Could you check a few things on this model? Use its own coordinates, in mm. A direction names the side the tool comes from. Coordinates: 2 decimals unless noted, no trailing zeros. Order: outer loops, then holes, each group sorted by start corner. A loop starts at its lowest first (then second) coordinate and runs counter-clockwise, first axis right, second up. Notation, with made-up numbers: (1.5, 14.5) - (49.5, 14.5) arc R26 ccw to (49.5, 36.5) - close; hole circle Ø10 at (33, 2). An arc over 180 degrees is marked (long way). Answer as a JSON object with one key per item and string values. Group by question number.
(1) Which directions (+Z, -Z, +X, -X, +Y, -Y) give clear straight access to the entire face, cutting with the end or side of a thin tool? Please do faces 1 (the cylindrical face through (68.57, 14.45, -7.45)), 2 (the flat face through (62, 22, -80)), 3 (the flat face through (9, 24, -11)), 4 (the flat face through (29, 40, -2)).
(2) Please list where these lines run through material, in increasing order: probe 1 along Y at (x, z) = (116, -8) (3 decimals); probe 2 along Y at (x, z) = (70, -10) (3 decimals); probe 3 along X at (y, z) = (26.5, -68.5).
(3) We'd pull the mould along X, two halves only. Please class faces 5 (the flat face through (0, 22, -39)), 6 (the flat face through (62, 22, 0)), 7 (the flat face through (121, 24, -39)): pulls with the +X half, pulls with the -X half, needs draft (parallel to the pull), parting line crosses it, or undercut.
(4) Imagine slicing it at C-C, the plane z = -44.5. Write out the boundary of the cut face in (x, y).
(5) Imagine slicing it at A-A, the plane y = 9.5. Write out the boundary of the cut face in (x, z), and give its area (3 significant figures).
(6) Imagine slicing it at B-B, the plane x = 77.5. Write out the boundary of the cut face in (y, z), and give its area (3 significant figures).
(7) Will these pins go through, and if not, where does the flat tip stop? P1, Ø4, axis at x = 63.5, z = -37, coming from the +Y side; P2, Ø4.5, axis at y = 24.5, z = -1.5, coming from the -X side.
from build123d import *

# Parameters (mm, degrees)
BASE_SKETCH_W                   = 125
BASE_SKETCH_H                   = 80
BASE_EXTRUDE_DEPTH              = 4
WALL_BASE_SKETCH_W              = 125
WALL_BASE_SKETCH_H              = 80
WALL_BASE_SKETCH_W_2            = 117
WALL_BASE_SKETCH_H_2            = 72
WALL_BASE_EXTRUDE_DEPTH         = 40
SPEAKER_HOLE_SKETCH_W           = 28
SPEAKER_HOLE_SKETCH_H           = 32
SPEAKER_HOLE_DEPTH              = 7
SPEAKER_STANDOFFS_SKETCH_R      = 3.5
SPEAKER_STANDOFFS_SKETCH_R_2    = 1.5
SPEAKER_STANDOFFS_EXTRUDE_DEPTH = 7
M1_2X0_25_TAPPED_HOLE2_D        = 0.95
M1_2X0_25_TAPPED_HOLE2_DEPTH    = 3.15
M1_2X0_25_TAPPED_HOLE2_TIP      = 0.285408794


with BuildPart() as part:
    # base sketch → base extrude (new body)
    with BuildSketch(Plane(origin=(0, 0, 0), x_dir=(1, 0, 0), z_dir=(0, 1, 0))):
        with Locations((62.5, 40)):
            Rectangle(BASE_SKETCH_W, BASE_SKETCH_H)
    extrude(amount=BASE_EXTRUDE_DEPTH)

    # wall base sketch → wall base extrude (add)
    with BuildSketch(Plane(origin=(0, 4, 0), x_dir=(1, 0, 0), z_dir=(0, 1, 0))):
        with Locations((62.5, 40)):
            Rectangle(WALL_BASE_SKETCH_W, WALL_BASE_SKETCH_H)
        with Locations((62.5, 40)):
            Rectangle(WALL_BASE_SKETCH_W_2, WALL_BASE_SKETCH_H_2, mode=Mode.SUBTRACT)
    extrude(amount=WALL_BASE_EXTRUDE_DEPTH)

    # speaker hole sketch → speaker hole (cut)
    with BuildSketch(Plane.XY):
        with Locations((29, 24)):
            Rectangle(SPEAKER_HOLE_SKETCH_W, SPEAKER_HOLE_SKETCH_H)
    extrude(amount=-SPEAKER_HOLE_DEPTH, mode=Mode.SUBTRACT)

    # speaker standoffs sketch → speaker standoffs extrude (add)
    with BuildSketch(Plane(origin=(0, 0, -4), x_dir=(-1, 0, 0), z_dir=(0, 0, -1))):
        with Locations((-48, 24)):
            Circle(SPEAKER_STANDOFFS_SKETCH_R)
        with Locations((-10, 24)):
            Circle(SPEAKER_STANDOFFS_SKETCH_R)
        with Locations((-116, 37)):
            Circle(SPEAKER_STANDOFFS_SKETCH_R_2)
        with Locations((-70, 37)):
            Circle(SPEAKER_STANDOFFS_SKETCH_R_2)
        with Locations((-116, 13.5)):
            Circle(SPEAKER_STANDOFFS_SKETCH_R_2)
        with Locations((-70, 14)):
            Circle(SPEAKER_STANDOFFS_SKETCH_R_2)
    extrude(amount=SPEAKER_STANDOFFS_EXTRUDE_DEPTH)

    # M1.2x0.25 Tapped Hole2
    with Locations(Plane(origin=(48, 24, -11), x_dir=(-1, 0, 0), z_dir=(0, 0, -1))):
        with Locations((0, 0), (38, 0), (-22, -10), (-22, 13), (-68, -10.5), (-68, 13)):
            Hole(M1_2X0_25_TAPPED_HOLE2_D / 2, depth=M1_2X0_25_TAPPED_HOLE2_DEPTH)
            with Locations((0, 0, -(M1_2X0_25_TAPPED_HOLE2_DEPTH + M1_2X0_25_TAPPED_HOLE2_TIP / 2))):  # 118° drill point
                Cone(0, M1_2X0_25_TAPPED_HOLE2_D / 2, M1_2X0_25_TAPPED_HOLE2_TIP, mode=Mode.SUBTRACT)


solid = part.part
Result set:
{
 "1": {"face 1": "none", "face 2": "-Z, +X, -X, +Y, -Y", "face 3": "+Y", "face 4": "+Z"},
 "2": {"probe 1": "y = 0 to 4, 12 to 13.025, 13.975 to 15, 35.5 to 36.525, 37.475 to 38.5", "probe 2": "y = 0 to 4, 12.5 to 13.525, 14.475 to 15.5, 35.5 to 36.525, 37.475 to 38.5", "probe 3": "x = 0 to 4, 121 to 125"},
 "3": {"face 5": "pulls with the -X half", "face 6": "needs draft", "face 7": "undercut"},
 "4": {"outline": "(0, 0) - (125, 0) - (125, 44) - (121, 44) - (121, 4) - (4, 4) - (4, 44) - (0, 44) - close"},
 "5": {"outline": "(0, -80) - (125, -80) - (125, 0) - (43, 0) - (43, -4) - (121, -4) - (121, -76) - (4, -76) - (4, -4) - (15, -4) - (15, 0) - (0, 0) - close", "area": "1,460 mm^2"},
 "6": {"outline": "(0, -80) - (44, -80) - (44, -76) - (4, -76) - (4, -4) - (44, -4) - (44, 0) - (0, 0) - close", "area": "640 mm^2"},
 "7": {"P1": "stops at y = 4", "P2": "stops at x = 0"}
}
